Study the drawing (mm; zero at the part's minimum x, y, z) and answer. Round coordinates to 2 decimals unless told otherwise and drop trailing zeros. Write each loop counter-clockwise with the first axis right and the second up, starting at its lowest first coordinate (ties: lowest second). Pieces come first, ordered by that corner, then holes. Notation, with made-up numbers: (42.5, 50) - (89.5, 50) arc R35 cw to (89.5, 89) - close; hole circle Ø3 at (45, 15.5). An arc over 180 degrees is marked (long way). Return JSON: item names as keys, results as strings. Group by question number.
(1) Section A-A, the plane y = 60 is taken. Write down the section's boundary in (x, z).
(2) Find the intervals of material crossed by line 1 along Y through (x, z) = (60, 18.5); line 2 along X through (y, z) = (77, 28.5); line 3 along Y through (x, z) = (52, 9), in increasing order. Write a range as [from, to].
(3) Section C-C, the plane z = 31 is taken. Write down the section's boundary in (x, y).
(4) Determine the mould class of the marked faces 1, 2, 3 and 4 for opening direction Y: +Y half, -Y half, draft (parallel to the pull), parting line (faces both ways), or undercut.
(5) This flat-tipped pin is pushed along its axis until it touches: pin 1 (12 mm diameter, centred on y = 19.5, z = 33.5, fed in from -X). Where does it stop, or does it pass through?
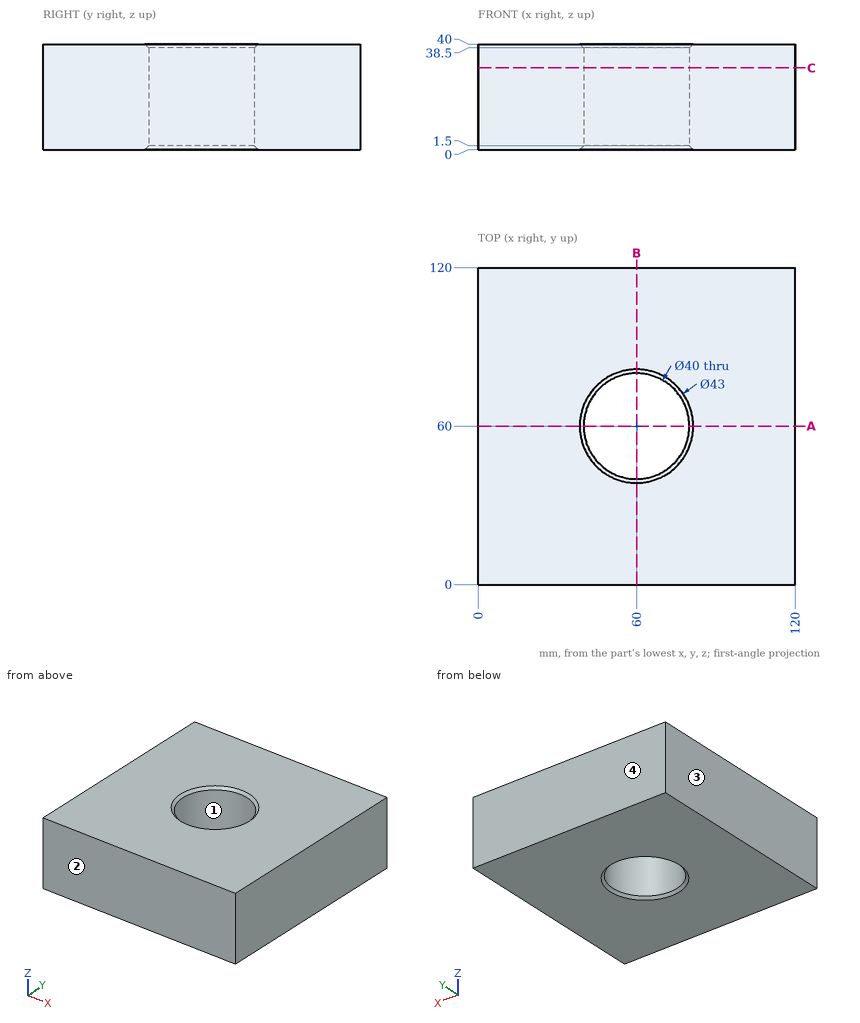
Working result:
{
 "1": {"outline": "(0, 0) - (38.5, 0) - (40, 1.5) - (40, 38.5) - (38.5, 40) - (0, 40) - close; (80, 1.5) - (81.5, 0) - (120, 0) - (120, 40) - (81.5, 40) - (80, 38.5) - close"},
 "2": {"line 1": "y = [0, 40], [80, 120]", "line 2": "x = [0, 49.46], [70.54, 120]", "line 3": "y = [0, 41.67], [78.33, 120]"},
 "3": {"outline": "(0, 0) - (120, 0) - (120, 120) - (0, 120) - close; hole circle Ø40 at (60, 60)"},
 "4": {"face 1": "undercut", "face 2": "-Y half", "face 3": "draft", "face 4": "+Y half"},
 "5": {"pin 1": "stops at x = 0"}
}
